Check sheet for the modelled part. Datum: model origin and axes. Units: mm. A direction names the side the tool comes from. Give positions to 0.01 mm unless a question says otherwise; leave off trailing zeros. Order: outer loops, then holes, each group sorted by start corner. A loop starts at its lowest first (then second) coordinate and runs counter-clockwise, first axis right, second up.
Item 1: Gauge pin test, flat ends, axial feed: P1, Ø8.5, axis at x = -35.5, y = -21, coming from the +Z side; P2, Ø1, axis at x = -27, z = -37, coming from the +Y side; P3, Ø10, axis at y = -52.5, z = 52.5, coming from the -X side. Record the tip position at first contact, or that the pin passes through.
Item 2: Access from +Z, -Z, +X, -X, +Y, -Y to the whole of each face (thin tool, end or side, straight path). Record for faces 1 (the flat face through (-34.203, -50.414, -77.535)), 2 (the cylindrical face through (-10.265, 7.098, -0.767)), 3 (the cylindrical face through (-27.9, -104.5, 27)), 4 (the conical face through (-34.203, -43.235, -70.527)).
Item 3: Sectioned sample at C-C on z = 22.5. Record the boundary of the cut face in (x, y), and give its area (3 significant figures).
Item 4: Sectioned sample at A-A on z = -67.3. Record the boundary of the cut face in (x, y).
Item 5: Sectioned sample at D-D on y = -31.5. Record the boundary of the cut face in (x, z), and give its area (3 significant figures).
Item 6: Sectioned sample at B-B on x = -12.5. Record the boundary of the cut face in (y, z).
Item 7: Release check for a two-part mould opening along Z. For faces 5 (the flat face through (-10, 0, 1)), 6 (the flat face through (-30.4, -52, 3)), 7 (the flat face through (-26, -28, 80)), 8 (the cylindrical face through (-27.935, -108.797, -78.859)) record: released by +Z, released by -Z, zero draft, split by the parting line, or undercut.
Item 8: Material ranges on line 1 along Z through (x, y) = (-30.5, -106) (3 decimals); line 2 along Z through (x, y) = (-29.75, 0); line 3 along Y through (x, z) = (-30.5, 75), recorded low to high.
from build123d import *

# Parameters (mm, degrees)
BOSS_EXTRUDE1_DEPTH                = 80
SKETCH2_R                          = 5
SKETCH2_R_2                        = 4
BOSS_EXTRUDE2_DEPTH                = 7.5
BOSS_EXTRUDE2_TAPER                = 7.8
CUT_EXTRUDE1_DEPTH                 = 31.4
CUT_EXTRUDE2_DEPTH                 = 31.4
SKETCH6_W                          = 4
SKETCH6_H                          = 43
SKETCH6_H_2                        = 49
EXTRUDE_THIN1_DEPTH                = 7.5
TAP_DRILL_FOR_M2_5X0_45_TAP1_D     = 2.05
TAP_DRILL_FOR_M2_5X0_45_TAP1_DEPTH = 10
TAP_DRILL_FOR_M2_5X0_45_TAP1_TIP   = 0.615882135
TAP_DRILL_FOR_M3X0_5_TAP1_D        = 2.5
TAP_DRILL_FOR_M3X0_5_TAP1_DEPTH    = 10
TAP_DRILL_FOR_M3X0_5_TAP1_TIP      = 0.751075774
BOSS_EXTRUDE4_DEPTH                = 160
F_10_CLEARANCE_HOLE1_D             = 5.1054


with BuildPart() as part:
    # Sketch1 → Boss-Extrude1 (new body, symmetric)
    with BuildSketch(Plane.XY):
        Polygon((0, 5), (-30.4, 5), (-30.4, -110), (-25.4, -110), (-25.4, 0), (0, 0), align=None)
    extrude(amount=BOSS_EXTRUDE1_DEPTH, both=True)

    # Sketch2 → Boss-Extrude2 (add)
    with BuildSketch(Plane.ZY.offset(30.4)):
        with Locations((75, -43)):
            Circle(SKETCH2_R)
        with Locations((75, 0)):
            Circle(SKETCH2_R)
        with Locations((-75, 0)):
            Circle(SKETCH2_R)
        with Locations((-75, -43)):
            Circle(SKETCH2_R)
        with Locations((-76, -57)):
            Circle(SKETCH2_R_2)
        with Locations((-76, -106)):
            Circle(SKETCH2_R_2)
        with Locations((-18, -106)):
            Circle(SKETCH2_R_2)
        with Locations((-18, -57)):
            Circle(SKETCH2_R_2)
    extrude(amount=BOSS_EXTRUDE2_DEPTH, taper=BOSS_EXTRUDE2_TAPER)

    # Sketch3 → Cut-Extrude1 (cut, through all)
    with BuildSketch(Plane.ZY.offset(30.4)):
        with BuildLine():
            Line((74, -56), (74, -102))
            ThreePointArc((74, -102), (72, -104), (70, -102))
            Line((70, -102), (70, -56))
            ThreePointArc((70, -56), (72, -54), (74, -56))
        make_face()
        with BuildLine():
            Line((55, -56.167316529), (55, -102.167316529))
            ThreePointArc((55, -102.167316529), (57, -104.167316529), (59, -102.167316529))
            Line((59, -102.167316529), (59, -56.167316529))
            ThreePointArc((59, -56.167316529), (57, -54.167316529), (55, -56.167316529))
        make_face()
        with BuildLine():
            Line((40, -56.334633058), (40, -102.334633058))
            ThreePointArc((40, -102.334633058), (42, -104.334633058), (44, -102.334633058))
            Line((44, -102.334633058), (44, -56.334633058))
            ThreePointArc((44, -56.334633058), (42, -54.334633058), (40, -56.334633058))
        make_face()
        with BuildLine():
            Line((25, -56.501949587), (25, -102.501949587))
            ThreePointArc((25, -102.501949587), (27, -104.501949587), (29, -102.501949587))
            Line((29, -102.501949587), (29, -56.501949587))
            ThreePointArc((29, -56.501949587), (27, -54.501949587), (25, -56.501949587))
        make_face()
        with BuildLine():
            Line((10, -56.669266116), (10, -102.669266116))
            ThreePointArc((10, -102.669266116), (12, -104.669266116), (14, -102.669266116))
            Line((14, -102.669266116), (14, -56.669266116))
            ThreePointArc((14, -56.669266116), (12, -54.669266116), (10, -56.669266116))
        make_face()
        with BuildLine():
            Line((-5, -56.836582645), (-5, -102.836582645))
            ThreePointArc((-5, -102.836582645), (-3, -104.836582645), (-1, -102.836582645))
            Line((-1, -102.836582645), (-1, -56.836582645))
            ThreePointArc((-1, -56.836582645), (-3, -54.836582645), (-5, -56.836582645))
        make_face()
    extrude(amount=-CUT_EXTRUDE1_DEPTH, mode=Mode.SUBTRACT)

    # Sketch4 → Cut-Extrude2 (cut, through all)
    with BuildSketch(Plane.ZY.offset(30.4)):
        with BuildLine():
            ThreePointArc((80, -106), (78.828427125, -108.828427125), (76, -110))
            Line((76, -110), (80, -110))
            Line((80, -110), (80, -106))
        make_face()
        with BuildLine():
            ThreePointArc((-80, -106), (-78.828427125, -108.828427125), (-76, -110))
            Line((-76, -110), (-80, -110))
            Line((-80, -110), (-80, -106))
        make_face()
    extrude(amount=-CUT_EXTRUDE2_DEPTH, mode=Mode.SUBTRACT)

    # Sketch6 → Extrude-Thin1 (add)
    with BuildSketch(Plane.ZY.offset(37.9)):
        Polygon((-74, -106), (-74, -57.071337695), (-73, -43.071337695), (-73, 0), (-77, 0), (-77, -42.928662305), (-78, -56.928662305), (-78, -106), align=None)
        with Locations((75, -21.5)):
            Rectangle(SKETCH6_W, SKETCH6_H)
        with Locations((-18, -81.5)):
            Rectangle(SKETCH6_W, SKETCH6_H_2)
    extrude(amount=-EXTRUDE_THIN1_DEPTH)

    # Tap Drill for M2.5x0.45 Tap1
    with Locations(Plane.ZY.offset(37.9)):
        with Locations((-76, -57), (-76, -106), (-18, -106), (-18, -57)):
            Hole(TAP_DRILL_FOR_M2_5X0_45_TAP1_D / 2, depth=TAP_DRILL_FOR_M2_5X0_45_TAP1_DEPTH)
            with Locations((0, 0, -(TAP_DRILL_FOR_M2_5X0_45_TAP1_DEPTH + TAP_DRILL_FOR_M2_5X0_45_TAP1_TIP / 2))):  # 118° drill point
                Cone(0, TAP_DRILL_FOR_M2_5X0_45_TAP1_D / 2, TAP_DRILL_FOR_M2_5X0_45_TAP1_TIP, mode=Mode.SUBTRACT)

    # Tap Drill for M3x0.5 Tap1
    with Locations(Plane(origin=(-37.9, 0, -75), x_dir=(0, -1, 0), z_dir=(-1, 0, 0))):
        with Locations((0, 0), (43, 0), (43, 150), (0, 150)):
            Hole(TAP_DRILL_FOR_M3X0_5_TAP1_D / 2, depth=TAP_DRILL_FOR_M3X0_5_TAP1_DEPTH)
            with Locations((0, 0, -(TAP_DRILL_FOR_M3X0_5_TAP1_DEPTH + TAP_DRILL_FOR_M3X0_5_TAP1_TIP / 2))):  # 118° drill point
                Cone(0, TAP_DRILL_FOR_M3X0_5_TAP1_D / 2, TAP_DRILL_FOR_M3X0_5_TAP1_TIP, mode=Mode.SUBTRACT)

    # Sketch11 → Boss-Extrude4 (add)
    with BuildSketch(Plane.XY.offset(80)):
        Polygon((-30.4, 5), (-21.4, 14), (0, 14), (0, 5), align=None)
    extrude(amount=-BOSS_EXTRUDE4_DEPTH)

    # #10 Clearance Hole1 (through all)
    with Locations(Plane(origin=(0, 0, 0), x_dir=(-1, 0, 0), z_dir=(0, -1, 0))):
        with Locations((12.7, 0), (12.7, 67.3), (12.7, -67.3)):
            Hole(F_10_CLEARANCE_HOLE1_D / 2)


solid = part.part
Report:
1. P1: stops at z = 77
1. P2: stops at y = 8.9
1. P3: stops at x = -30.4
2. face 1: -Z, -X
2. face 2: +Y, -Y
2. face 3: +X, -X
2. face 4: -X
3. outline: (-30.4, -110) - (-25.4, -110) - (-25.4, 0) - (0, 0) - (0, 14) - (-21.4, 14) - (-30.4, 5) - close
3. area: 935 mm2
4. outline: (-30.4, -110) - (-25.4, -110) - (-25.4, 0) - (-15.25, 0) - (-15.25, 14) - (-21.4, 14) - (-30.4, 5) - close; (-10.15, 0) - (0, 0) - (0, 14) - (-10.15, 14) - close
5. outline: (-37.9, -77) - (-30.4, -77) - (-30.4, -80) - (-25.4, -80) - (-25.4, 80) - (-30.4, 80) - (-30.4, 77) - (-37.9, 77) - (-37.9, 73) - (-30.4, 73) - (-30.4, -73) - (-37.9, -73) - close
5. area: 860 mm2
6. outline: (0, -80) - (14, -80) - (14, -69.84) - (0, -69.84) - close; (0, -64.76) - (14, -64.76) - (14, -2.54) - (0, -2.54) - close; (0, 2.54) - (14, 2.54) - (14, 64.76) - (0, 64.76) - close; (0, 69.84) - (14, 69.84) - (14, 80) - (0, 80) - close
7. face 5: zero draft
7. face 6: undercut
7. face 7: released by +Z
7. face 8: released by -Z
8. line 1: z = -79.986 to -77.025, -74.975 to -72.014, -21.986 to -19.025, -16.975 to -14.014
8. line 2: z = -80 to -76.25, -73.75 to 73.75, 76.25 to 80
8. line 3: y = -47.99 to -44.25, -41.75 to -1.25, 1.25 to 4.99
